Source: three-view drawing plus pictorial views. Frame: mm from the lowest corner of the part. A direction names the side the tool comes from. Give positions to 0.01 mm unless a question says otherwise; leave off trailing zeros. Loops run counter-clockwise (first coordinate to the right, second up) from the corner with the lowest first, then second, coordinate; pieces in that order, holes last. Notation, with made-up numbers: (14.5, 35) - (18.5, 35) arc R16 cw to (18.5, 66) - close; hole circle Ø4 at (-23, -22). An arc over 180 degrees is marked (long way). Answer as a JSON object with one key per item and string values.
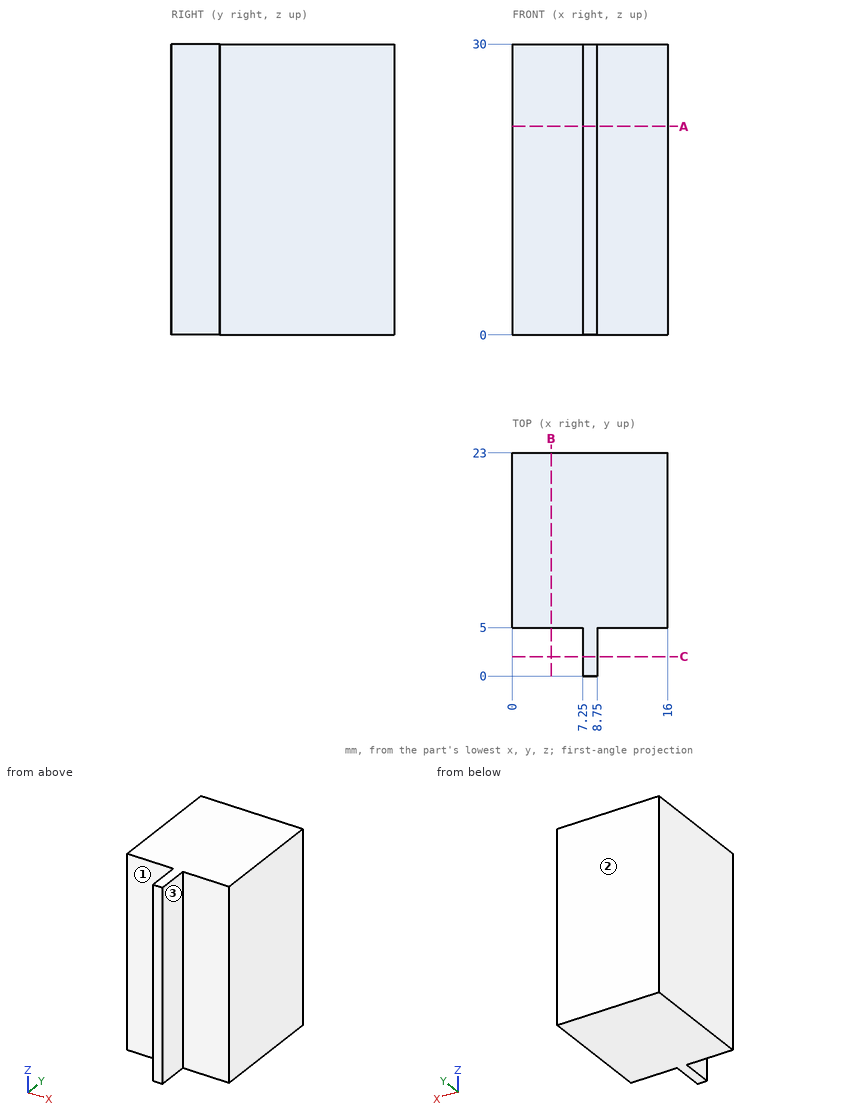
Item 1: Contact query for flat-ended pins moving along their axis: P1, Ø8, axis at x = 3, z = 15.5, coming from the -Y side; P2, Ø5.5, axis at y = 2, z = 14.5, coming from the -X side. Output: stop coordinate, or through.
Geometry check:
{"P1": "stops at y = 5", "P2": "stops at x = 7.25"}
Item 2: Material intervals for line 1 (Y direction, x = 3.5, z = 18.5); line 2 (X direction, y = 4.5, z = 24.5), sorted ascending. Write a range as [from, to].
Geometry check:
{"line 1": "y = [5, 23]", "line 2": "x = [7.25, 8.75]"}
Item 3: Cut plane C-C (y = 2). Return loops of the section in (x, z), then the cut area to 3 significant figures.
Geometry check:
{"outline": "(7.25, 0) - (8.75, 0) - (8.75, 30) - (7.25, 30) - close", "area": "45.0 mm2"}
Item 4: Cut plane A-A (z = 21.5). Return loops of the section in (x, y), then the cut area to 4 significant figures.
Geometry check:
{"outline": "(0, 5) - (7.25, 5) - (7.25, 0) - (8.75, 0) - (8.75, 5) - (16, 5) - (16, 23) - (0, 23) - close", "area": "295.5 mm2"}
Item 5: Cut plane B-B (x = 4). Return loops of the section in (y, z).
Geometry check:
{"outline": "(5, 0) - (23, 0) - (23, 30) - (5, 30) - close"}
Item 6: Access query for the marked faces 1, 2 and 3. Directions: +Z, -Z, +X, -X, +Y, -Y. A direction counts if a zero-diameter tool reaches every point of the face in a straight line with its end or side. Return the directions, or none.
Geometry check:
{"face 1": "+Z, -Z, -X, -Y", "face 2": "+Z, -Z, +X, -X, +Y", "face 3": "+Z, -Z, +X, -Y"}
